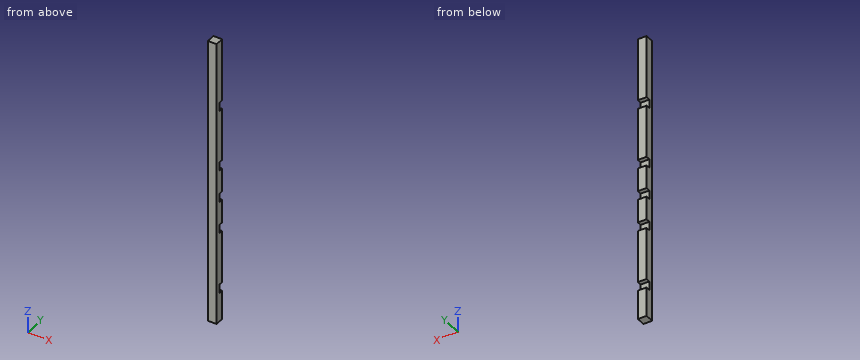
```python
from build123d import *

# Parameters (mm, degrees)
F1_DEPTH = 19.05
F0_W     = 228.6
F0_H     = 38.1
F0_W_2   = 273.05
F0_W_3   = 101.6
F0_W_4   = 127
F2_W     = 1250.95
F2_H     = 38.1
F3_DEPTH = 19.05
F5_ANGLE = 90
F6_ANGLE = 90


with BuildPart() as f1:
    # F0 (on Top) → F1 (new body)
    with BuildSketch(Plane.XY):
        Polygon((-50.8, 0), (0, 0), (50.8, 0), (50.8, 38.1), (-50.8, 38.1), align=None)
    extrude(amount=F1_DEPTH)


with BuildPart() as f1b:
    # F0 (on Top) → F1, piece 2 (new body)
    with BuildSketch(Plane.XY):
        with Locations((203.2, 19.05)):
            Rectangle(F0_W, F0_H)
    extrude(amount=F1_DEPTH)


with BuildPart() as f1c:
    # F0 (on Top) → F1, piece 3 (new body)
    with BuildSketch(Plane.XY):
        with Locations((492.125, 19.05)):
            Rectangle(F0_W_2, F0_H)
    extrude(amount=F1_DEPTH)


with BuildPart() as f1d:
    # F0 (on Top) → F1, piece 4 (new body)
    with BuildSketch(Plane.XY):
        with Locations((-139.7, 19.05)):
            Rectangle(F0_W_3, F0_H)
    extrude(amount=F1_DEPTH)


with BuildPart() as f1e:
    # F0 (on Top) → F1, piece 5 (new body)
    with BuildSketch(Plane.XY):
        with Locations((-342.9, 19.05)):
            Rectangle(F0_W, F0_H)
    extrude(amount=F1_DEPTH)


with BuildPart() as f1f:
    # F0 (on Top) → F1, piece 6 (new body)
    with BuildSketch(Plane.XY):
        with Locations((-558.8, 19.05)):
            Rectangle(F0_W_4, F0_H)
    extrude(amount=F1_DEPTH)


with BuildPart() as f3:
    # F2 (on face) → F3 (new body)
    with BuildSketch(Plane.XY.offset(19.05)):
        with Locations((3.175, 19.05)):
            Rectangle(F2_W, F2_H)
    extrude(amount=F3_DEPTH)

    # F4: union F1, F1b, F1c, F1d, F1e, F1f
    add(f1.part)
    add(f1b.part)
    add(f1c.part)
    add(f1d.part)
    add(f1e.part)
    add(f1f.part)


with BuildPart() as f3_1:
    # F5: moved
    add(f3.part.rotate(Axis((-622.3, 19.05, 38.1), (0, -1, 0)), F5_ANGLE))


with BuildPart() as f3_2:
    # F6: moved
    add(f3_1.part.rotate(Axis((-622.3, 38.1, 663.575), (0, 0, 1)), F6_ANGLE))


solid = f3_2.part
```
Build history of the part. All positions in model axes, mm. Round coordinates to 2 decimals unless told otherwise and drop trailing zeros. Write each loop counter-clockwise with the first axis right and the second up, starting at its lowest first coordinate (ties: lowest second). Pieces come first, ordered by that corner, then holes.
1) Band-saw the part on C-C, the plane z = 443.5. List the corners of the cut face in (x, y), and give its area (3 significant figures).
2) Drill centre lines: probe 1 along Z at (x, y) = (-610.5, 64.5); probe 2 along Y at (x, z) = (-598.5, 451). Where is each one in solid material? Low to high.
3) Band-saw the part on B-B, the plane x = -606. List the corners of the cut face in (y, z), and give its area (3 significant figures).
4) Band-saw the part on A-A, the plane y = 68. List the corners of the cut face in (x, z), and give its area (3 significant figures).
5) Pin check, flat tip, straight feed: pin 1 (19 mm diameter, centred on x = -603, z = 587, fed in from +Y). Stop position of the tip, or through.
Ans:
1. outline: (-622.3, 38.1) - (-584.2, 38.1) - (-584.2, 57.15) - (-622.3, 57.15) - close
1. area: 726 mm2
2. probe 1: z = 38.1 to 165.1, 203.2 to 431.8, 469.9 to 571.5, 609.6 to 711.2, 749.3 to 977.9, 1016 to 1289.05
2. probe 2: y = 38.1 to 57.15
3. outline: (38.1, 38.1) - (76.2, 38.1) - (76.2, 165.1) - (57.15, 165.1) - (57.15, 203.2) - (76.2, 203.2) - (76.2, 431.8) - (57.15, 431.8) - (57.15, 469.9) - (76.2, 469.9) - (76.2, 571.5) - (57.15, 571.5) - (57.15, 609.6) - (76.2, 609.6) - (76.2, 711.2) - (57.15, 711.2) - (57.15, 749.3) - (76.2, 749.3) - (76.2, 977.9) - (57.15, 977.9) - (57.15, 1016) - (76.2, 1016) - (76.2, 1289.05) - (38.1, 1289.05) - close
3. area: 44,000 mm2
4. outline: (-622.3, 38.1) - (-584.2, 38.1) - (-584.2, 165.1) - (-622.3, 165.1) - close; (-622.3, 203.2) - (-584.2, 203.2) - (-584.2, 431.8) - (-622.3, 431.8) - close; (-622.3, 469.9) - (-584.2, 469.9) - (-584.2, 571.5) - (-622.3, 571.5) - close; (-622.3, 609.6) - (-584.2, 609.6) - (-584.2, 711.2) - (-622.3, 711.2) - close; (-622.3, 749.3) - (-584.2, 749.3) - (-584.2, 977.9) - (-622.3, 977.9) - close; (-622.3, 1016) - (-584.2, 1016) - (-584.2, 1289.05) - (-622.3, 1289.05) - close
4. area: 40,400 mm2
5. pin 1: stops at y = 57.15
